Autodesk Fusion 360 part; units mm, degrees
sketch "Sketch1" plane through (0, 0, 0) normal (1, 0, 0) x (0, 1, 0)
  circle A0 centre (0, 0) radius 4.5
  dimension "d1" = 9
extrude "Extrude1" add sketch "Sketch1" along normal mid plane 44
sketch "Sketch3" plane through (0, 0, 0) normal (1, 0, 0) x (0, 1, 0)
  circle A0 centre (0, 0) radius 4
  circle A1 centre (0, 0) radius 5
  dimension "d7" = 8
  dimension "d8" = 10
extrude "Extrude2" cut sketch "Sketch3" along normal mid plane 36
The listing builds one solid part. Answer for the finished solid, in the listing's coordinates (mm). A direction names the side the tool comes from. Coordinates: 2 decimals unless noted, no trailing zeros. Write each loop counter-clockwise with the first axis right and the second up, starting at its lowest first coordinate (ties: lowest second). Pieces come first, ordered by that corner, then holes. Notation, with made-up numbers: (14.25, -26) - (63.25, -26) arc R29 cw to (63.25, -2) - close; hole circle Ø1 at (62.5, -35.75). An arc over 180 degrees is marked (long way). Return JSON: item names as keys, results as strings.
1. The part is cut by section A-A on y = 0. Determine the outline of the cut face in (x, z), then the cut area to 3 significant figures.
Final values:
{"outline": "(-22, -4.5) - (-18, -4.5) - (-18, -4) - (18, -4) - (18, -4.5) - (22, -4.5) - (22, 4.5) - (18, 4.5) - (18, 4) - (-18, 4) - (-18, 4.5) - (-22, 4.5) - close", "area": "360 mm^2"}
2. Consider line 1 along X through (y, z) = (-3.75, 1.75); line 2 along Z through (x, y) = (-13.5, -0.25); line 3 along Z through (x, y) = (13.5, 2.75). Determine where each line is inside the solid, lowest interval first.
Final values:
{"line 1": "-22 to -18, 18 to 22", "line 2": "-3.99 to 3.99", "line 3": "-2.9 to 2.9"}
3. For a pull along X with two mould halves and no side action, classify faces 3 (the face through (-19.97, -0.59, 4.46)), 4 (the face through (22, 0, 0)), 5 (the face through (18, -3, -3)), 6 (the face through (0.252, -0.867, -3.905)) as +X half, -X half, draft (parallel to the pull), parting line (faces both ways), or undercut.
Final values:
{"face 3": "draft", "face 4": "+X half", "face 5": "undercut", "face 6": "undercut"}
4. Which of the six approach directions +Z, -Z, +X, -X, +Y, -Y give full straight-line access (tool end or side, diameter ignored) to faces 1 (the face through (-18, -3, -3)), 2 (the face through (19.97, -0.59, -4.46))?
Final values:
{"face 1": "none", "face 2": "+X, -X"}
5. The part is cut by section C-C on x = 0. Determine the outline of the cut face in (y, z).
Final values:
{"outline": "circle Ø8 at (0, 0)"}
6. Each of these flat-tipped pins is pushed along its axis until it touches: pin 1 Ø2 at (x, y) = (-15, 0.5) entering from +Z; pin 2 Ø1.5 at (x, y) = (11, -2.5) entering from +Z; pin 3 Ø4 at (x, y) = (-16, -3.5) entering from +Z. Where does it stop, or does it pass through?
Final values:
{"pin 1": "z = 4", "pin 2": "z = 3.6", "pin 3": "z = 3.71"}
7. The part is cut by section D-D on x = -18.5. Determine the outline of the cut face in (y, z), then the cut area to 3 significant figures.
Final values:
{"outline": "circle Ø9 at (0, 0)", "area": "63.6 mm^2"}
